```python
from build123d import *

# Parameters (mm, degrees)
CROQUIS1_W              = 65
CROQUIS1_H              = 35
SALIENTE_EXTRUIR1_DEPTH = 2.5
CHAMFER1_SIZE           = 2
BOSS_EXTRUDE1_START     = -2.5
BOSS_EXTRUDE1_DEPTH     = 1.5
CHAMFER2_SIZE           = 1.5
CHAMFER2_SIZE_2         = 0.1
SKETCH2_W               = 1.1
SKETCH2_H               = 2.1
CUT_EXTRUDE1_DEPTH      = 0.6


with BuildPart() as part:
    # Croquis1 → Saliente-Extruir1 (new body)
    with BuildSketch(Plane.XY):
        Rectangle(CROQUIS1_W, CROQUIS1_H)
    extrude(amount=SALIENTE_EXTRUIR1_DEPTH)

    # Chamfer1
    chamfer1_edges = [part.edges().sort_by_distance(p)[0] for p in [
        (-32.5, 17.5, 1.25),
        (-32.5, -17.5, 1.25),
        (32.5, -17.5, 1.25),
        (32.5, 17.5, 1.25),
    ]]
    chamfer(chamfer1_edges, length=CHAMFER1_SIZE)

    # Sketch1 → Boss-Extrude1 (add)
    with BuildSketch(Plane.XY.offset(2.5).offset(BOSS_EXTRUDE1_START)):
        Polygon((-30.085786438, -16.5), (30.085786438, -16.5), (31.5, -15.085786438), (31.5, 15.085786438), (30.085786438, 16.5), (-30.085786438, 16.5), (-31.5, 15.085786438), (-31.5, -15.085786438), align=None)
        Polygon((-29.671572875, -15.5), (29.671572875, -15.5), (30.5, -14.671572875), (30.5, 14.671572875), (29.671572875, 15.5), (-29.671572875, 15.5), (-30.5, 14.671572875), (-30.5, -14.671572875), align=None, mode=Mode.SUBTRACT)
    extrude(amount=-BOSS_EXTRUDE1_DEPTH)

    # Chamfer2
    # the kernel refuses this chamfer: 1.5, 0.1 mm, written as the material it takes off along each edge
    with BuildSketch(Plane(origin=(34.257490553, 12.328295884, -1.5), x_dir=(0.0018092267925963327, 0.001809226792596321, 0.9999967266930556), z_dir=(-0.7071067811865454, 0.7071067811865498, 0))) as chamfer2_piece_1_section:
        Polygon((CHAMFER2_SIZE * 0.999996726693, -CHAMFER2_SIZE * 0.0025586330675), (-CHAMFER2_SIZE_2 * 0.0025586330675, -CHAMFER2_SIZE_2 * 0.999996726693), (0, 0), align=None)
    chamfer2_piece_1 = extrude(amount=9.799361077, mode=Mode.PRIVATE)
    chamfer2_piece_1 = split(chamfer2_piece_1, bisect_by=Plane(origin=(30.78142094, 15.78142094, 0), z_dir=(0, 0, -1)), keep=Keep.TOP, mode=Mode.PRIVATE)
    add(chamfer2_piece_1, mode=Mode.SUBTRACT)
    with BuildSketch(Plane(origin=(33.985466976, 16.5, -1.5), x_dir=(0, 0.0025586330674999794, 0.9999967266930556), z_dir=(-1, 0, 0))) as chamfer2_piece_2_section:
        Polygon((CHAMFER2_SIZE * 0.999996726693, -CHAMFER2_SIZE * 0.0025586330675), (-CHAMFER2_SIZE_2 * 0.0025586330675, -CHAMFER2_SIZE_2 * 0.999996726693), (0, 0), align=None)
    chamfer2_piece_2 = extrude(amount=67.970933952, mode=Mode.PRIVATE)
    chamfer2_piece_2 = split(chamfer2_piece_2, bisect_by=Plane(origin=(0, 16.483775747, 0), z_dir=(0, 0, -1)), keep=Keep.TOP, mode=Mode.PRIVATE)
    add(chamfer2_piece_2, mode=Mode.SUBTRACT)
    with BuildSketch(Plane(origin=(-27.328295884, 19.257490553, -1.5), x_dir=(-0.0018092267925980316, 0.0018092267925980384, 0.9999967266930556), z_dir=(-0.7071067811865489, -0.7071067811865462, 0))) as chamfer2_piece_3_section:
        Polygon((CHAMFER2_SIZE * 0.999996726693, -CHAMFER2_SIZE * 0.0025586330675), (-CHAMFER2_SIZE_2 * 0.0025586330675, -CHAMFER2_SIZE_2 * 0.999996726693), (0, 0), align=None)
    chamfer2_piece_3 = extrude(amount=9.799361077, mode=Mode.PRIVATE)
    chamfer2_piece_3 = split(chamfer2_piece_3, bisect_by=Plane(origin=(-30.78142094, 15.78142094, 0), z_dir=(0, 0, -1)), keep=Keep.TOP, mode=Mode.PRIVATE)
    add(chamfer2_piece_3, mode=Mode.SUBTRACT)
    with BuildSketch(Plane(origin=(-31.5, 18.985466976, -1.5), x_dir=(-0.0025586330674999794, 0, 0.9999967266930556), z_dir=(0, -1, 0))) as chamfer2_piece_4_section:
        Polygon((CHAMFER2_SIZE * 0.999996726693, -CHAMFER2_SIZE * 0.0025586330675), (-CHAMFER2_SIZE_2 * 0.0025586330675, -CHAMFER2_SIZE_2 * 0.999996726693), (0, 0), align=None)
    chamfer2_piece_4 = extrude(amount=37.970933952, mode=Mode.PRIVATE)
    chamfer2_piece_4 = split(chamfer2_piece_4, bisect_by=Plane(origin=(-31.483775747, 0, 0), z_dir=(0, 0, -1)), keep=Keep.TOP, mode=Mode.PRIVATE)
    add(chamfer2_piece_4, mode=Mode.SUBTRACT)
    with BuildSketch(Plane(origin=(-34.257490553, -12.328295884, -1.5), x_dir=(-0.0018092267925951928, -0.0018092267925951832, 0.9999967266930556), z_dir=(0.7071067811865458, -0.7071067811865493, 0))) as chamfer2_piece_5_section:
        Polygon((CHAMFER2_SIZE * 0.999996726693, -CHAMFER2_SIZE * 0.0025586330675), (-CHAMFER2_SIZE_2 * 0.0025586330675, -CHAMFER2_SIZE_2 * 0.999996726693), (0, 0), align=None)
    chamfer2_piece_5 = extrude(amount=9.799361077, mode=Mode.PRIVATE)
    chamfer2_piece_5 = split(chamfer2_piece_5, bisect_by=Plane(origin=(-30.78142094, -15.78142094, 0), z_dir=(0, 0, -1)), keep=Keep.TOP, mode=Mode.PRIVATE)
    add(chamfer2_piece_5, mode=Mode.SUBTRACT)
    with BuildSketch(Plane(origin=(31.5, -18.985466976, -1.5), x_dir=(0.0025586330674999794, 0, 0.9999967266930556), z_dir=(0, 1, 0))) as chamfer2_piece_6_section:
        Polygon((CHAMFER2_SIZE * 0.999996726693, -CHAMFER2_SIZE * 0.0025586330675), (-CHAMFER2_SIZE_2 * 0.0025586330675, -CHAMFER2_SIZE_2 * 0.999996726693), (0, 0), align=None)
    chamfer2_piece_6 = extrude(amount=37.970933952, mode=Mode.PRIVATE)
    chamfer2_piece_6 = split(chamfer2_piece_6, bisect_by=Plane(origin=(31.483775747, 0, 0), z_dir=(0, 0, -1)), keep=Keep.TOP, mode=Mode.PRIVATE)
    add(chamfer2_piece_6, mode=Mode.SUBTRACT)
    with BuildSketch(Plane(origin=(27.328295884, -19.257490553, -1.5), x_dir=(0.0018092267925980349, -0.0018092267925980349, 0.9999967266930556), z_dir=(0.7071067811865476, 0.7071067811865476, 0))) as chamfer2_piece_7_section:
        Polygon((CHAMFER2_SIZE * 0.999996726693, -CHAMFER2_SIZE * 0.0025586330675), (-CHAMFER2_SIZE_2 * 0.0025586330675, -CHAMFER2_SIZE_2 * 0.999996726693), (0, 0), align=None)
    chamfer2_piece_7 = extrude(amount=9.799361077, mode=Mode.PRIVATE)
    chamfer2_piece_7 = split(chamfer2_piece_7, bisect_by=Plane(origin=(30.78142094, -15.78142094, 0), z_dir=(0, 0, -1)), keep=Keep.TOP, mode=Mode.PRIVATE)
    add(chamfer2_piece_7, mode=Mode.SUBTRACT)
    with BuildSketch(Plane(origin=(-33.985466976, -16.5, -1.5), x_dir=(0, -0.0025586330674999794, 0.9999967266930556), z_dir=(1, 0, 0))) as chamfer2_piece_8_section:
        Polygon((CHAMFER2_SIZE * 0.999996726693, -CHAMFER2_SIZE * 0.0025586330675), (-CHAMFER2_SIZE_2 * 0.0025586330675, -CHAMFER2_SIZE_2 * 0.999996726693), (0, 0), align=None)
    chamfer2_piece_8 = extrude(amount=67.970933952, mode=Mode.PRIVATE)
    chamfer2_piece_8 = split(chamfer2_piece_8, bisect_by=Plane(origin=(0, -16.483775747, 0), z_dir=(0, 0, -1)), keep=Keep.TOP, mode=Mode.PRIVATE)
    add(chamfer2_piece_8, mode=Mode.SUBTRACT)

    # Sketch2 → Cut-Extrude1 (cut)
    with BuildSketch(Plane(origin=(0, 0, 0), x_dir=(-1, 0, 0), z_dir=(0, 0, -1))):
        with Locations((-31.5, 0)):
            Rectangle(SKETCH2_W, SKETCH2_H)
        with Locations((31.5, 0)):
            Rectangle(SKETCH2_W, SKETCH2_H)
    extrude(amount=CUT_EXTRUDE1_DEPTH, mode=Mode.SUBTRACT)


solid = part.part
```
Input: part model. Units: mm. Frame: model coordinates. A direction names the side the tool comes from. Give positions to 0.01 mm unless a question says otherwise; leave off trailing zeros. Order: outer loops, then holes, each group sorted by start corner. A loop starts at its lowest first (then second) coordinate and runs counter-clockwise, first axis right, second up.
1. Section B-B on x = -17.5. Return the cut outline in (y, z).
Derived:
outline: (-17.5, 0) - (-16.5, 0) - (-16.4, -1.5) - (-15.5, -1.5) - (-15.5, 0) - (15.5, 0) - (15.5, -1.5) - (16.4, -1.5) - (16.5, 0) - (17.5, 0) - (17.5, 2.5) - (-17.5, 2.5) - close
2. Material intervals for L1, parallel to X at y = 0, z = -1.3; L2, parallel to X at y = 0, z = -0.1; L3, parallel to Y at x = 27, z = -1.3, sorted ascending.
Derived:
L1: x = -31.41 to -30.5, 30.5 to 31.41
L2: x = -30.95 to -30.5, 30.5 to 30.95
L3: y = -16.41 to -15.5, 15.5 to 16.41
3. Reachability of faces 4 (the flat face through (30.748, -15.768, -0.739)), 5 (the flat face through (0, 0, 0)) from +Z, -Z, +X, -X, +Y, -Y: full face, straight path, thin tool, end or side. Return the list, or none.
Derived:
face 4: -Z, +X, -Y
face 5: -Z
4. Section A-A on y = -2.5. Return the cut outline in (x, z).
Derived:
outline: (-32.5, 0) - (-31.5, 0) - (-31.4, -1.5) - (-30.5, -1.5) - (-30.5, 0) - (30.5, 0) - (30.5, -1.5) - (31.4, -1.5) - (31.5, 0) - (32.5, 0) - (32.5, 2.5) - (-32.5, 2.5) - close
5. Mould query, pull axis X, two halves, no side actions, for faces 1 (the flat face through (0, -15.5, -1)), 2 (the flat face through (32, -16, 1)), 3 (the flat face through (0, 0, 2.5)). Classes: released by +X, released by -X, zero draft, split by the parting line, or undercut.
Derived:
face 1: undercut
face 2: released by +X
face 3: zero draft
6. Pin query (flat end, axial travel): pin 1 (1.2 mm diameter, centred on y = 6.5, z = -1, fed in from -X); pin 2 (6 mm diameter, centred on x = 0, y = 3.5, fed in from -Z); pin 3 (0.8 mm diameter, centred on x = 2, z = -0.5, fed in from -Y). Return the tip coordinate at first contact, or that it passes through.
Derived:
pin 1: stops at x = -31.47
pin 2: stops at z = 0
pin 3: stops at y = -16.49
